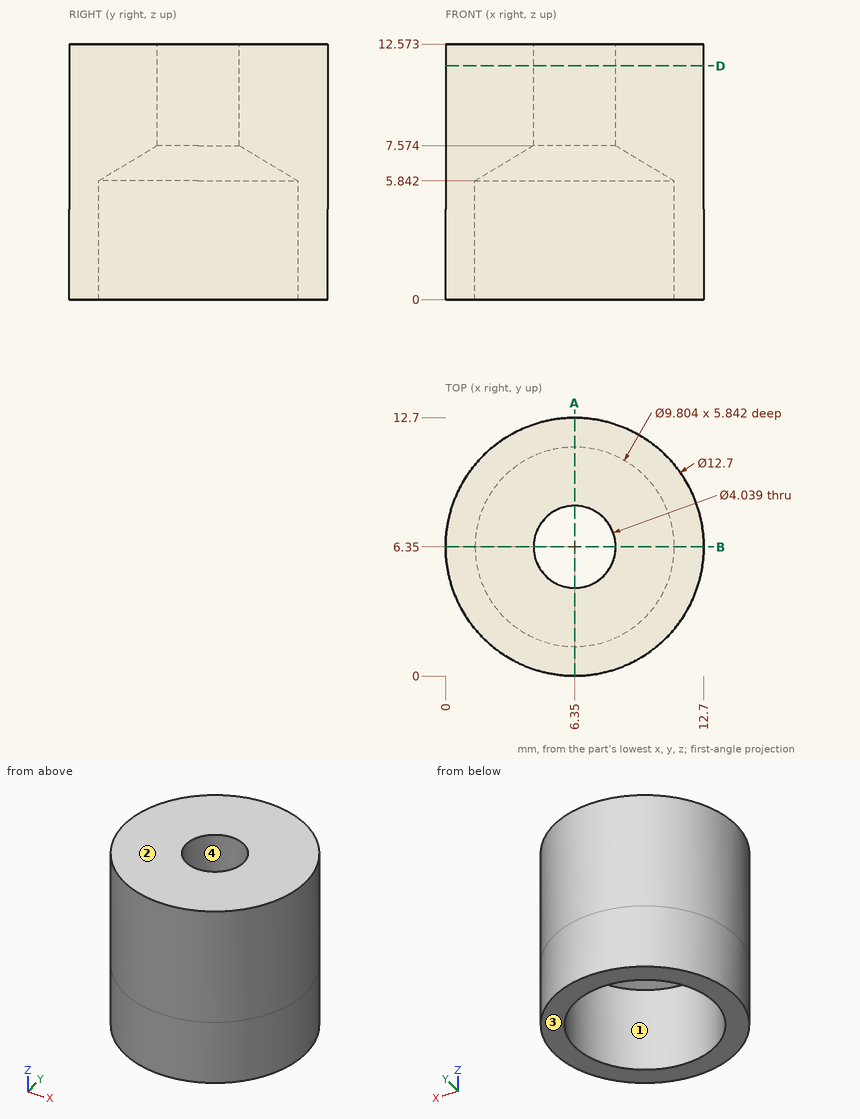
Can you work these out from the drawing? Everything is in mm from the part's minimum corner. A direction names the side the tool comes from. Give positions to 0.01 mm unless a question says otherwise; leave off trailing zeros. Order: outer loops, then holes, each group sorted by start corner. A loop starts at its lowest first (then second) coordinate and runs counter-clockwise, first axis right, second up. Notation, with made-up numbers: M -38,-16 L 9,-16 A29 cw 9,15 Z; hole C -9,1.25 d7. An arc over 180 degrees is marked long. One line per item, written item: value.
Item 1: If we mould it in two halves opening along Y, with no side actions, what happens to the marked faces 3 and 4? For each: pulls with the +Y half, pulls with the -Y half, needs draft (parallel to the pull), parting line crosses it, or undercut.
Verdict:
face 3: needs draft
face 4: undercut
Item 2: For the marked faces 1 and 2, which set-ups out of +Z, -Z, +X, -X, +Y, -Y let a thin tool reach every point of the face, with its end or its side?
Verdict:
face 1: -Z
face 2: +Z, +X, -X, +Y, -Y
Item 3: For pin 1 (6 mm diameter, centred on x = 11.5, z = 8, fed in from -Y) (1 decimal); pin 2 (6 mm diameter, centred on x = 6.35, y = 6.35, fed in from -Z) (1 decimal); pin 3 (2 mm diameter, centred on y = 11, z = 9.5, fed in from -X) (1 decimal), each with a flat end and sliding along its axis, tell me the tip position at first contact or that it passes through.
Verdict:
pin 1: y = 0.4
pin 2: z = 7
pin 3: x = 1.2
Item 4: Please list where these lines run through material, in increasing order: line 1 (Y direction, x = 6.35, z = 11.45); line 2 (Y direction, x = 6.35, z = 3.1); line 3 (X direction, y = 9.5, z = 5.75) (1 decimal).
Verdict:
line 1: 0 to 4.33, 8.37 to 12.7
line 2: 0 to 1.45, 11.25 to 12.7
line 3: 0.8 to 2.6, 10.1 to 11.9
Item 5: If we section it at A-A on x = 6.35: Write out the boundary of the cut face in (y, z) (1 decimal).
Verdict:
outline: M 0,0 L 1.4,0 L 1.4,5.8 L 4.3,7.6 L 4.3,12.6 L 0,12.6 Z; M 8.4,7.6 L 11.3,5.8 L 11.3,0 L 12.7,0 L 12.7,12.6 L 8.4,12.6 Z
Item 6: If we section it at D-D on z = 11.5: Write out the boundary of the cut face in (x, y).
Verdict:
outline: C 6.35,6.35 d12.7; hole C 6.35,6.35 d4.04
